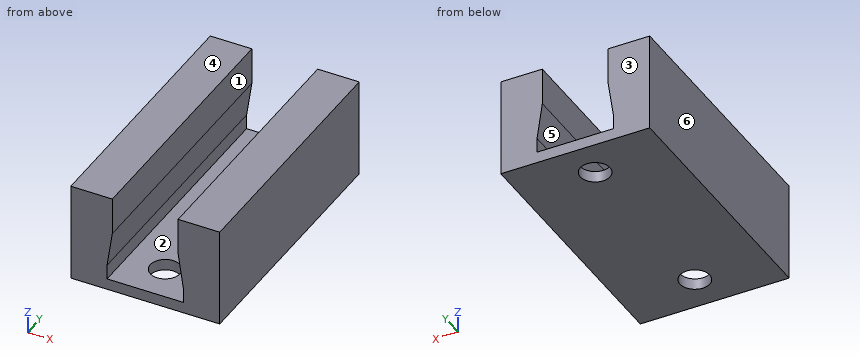
```python
from build123d import *

# Parameters (mm, degrees)
F1_DEPTH = 35
F2_R     = 2
F3_DEPTH = 8.301
F8_DEPTH = 35.001
F9_DEPTH = 5


# Not quite as in the source:
# - a feature names something its author has since deleted; it is built from what else it names


with BuildPart() as f1:
    # F0 (on Front) → F1 (new body)
    with BuildSketch(Plane.XZ):
        Polygon((10, 4.15), (4.15, 4.15), (-4.15, 4.15), (-10, 4.15), (-10, -4.15), (-4.15, -4.15), (4.15, -4.15), (10, -4.15), align=None)
        with BuildLine():
            ThreePointArc((5.15, -1.65), (4.8571067812, -2.3571067812), (4.15, -2.65))
            Line((4.15, -2.65), (-4.15, -2.65))
            ThreePointArc((-4.15, -2.65), (-4.8571067812, -2.3571067812), (-5.15, -1.65))
            Line((-5.15, -1.65), (-5.15, 1.65))
            ThreePointArc((-5.15, 1.65), (-4.8571067812, 2.3571067812), (-4.15, 2.65))
            Line((-4.15, 2.65), (4.15, 2.65))
            ThreePointArc((4.15, 2.65), (4.8571067812, 2.3571067812), (5.15, 1.65))
            Line((5.15, 1.65), (5.15, -1.65))
        make_face(mode=Mode.SUBTRACT)
        with BuildLine():
            Line((-4.15, -2.65), (4.15, -2.65))
            ThreePointArc((4.15, -2.65), (4.8571067812, -2.3571067812), (5.15, -1.65))
            Line((5.15, -1.65), (5.15, 1.65))
            ThreePointArc((5.15, 1.65), (4.8571067812, 2.3571067812), (4.15, 2.65))
            Line((4.15, 2.65), (-4.15, 2.65))
            ThreePointArc((-4.15, 2.65), (-4.8571067812, 2.3571067812), (-5.15, 1.65))
            Line((-5.15, 1.65), (-5.15, -1.65))
            ThreePointArc((-5.15, -1.65), (-4.8571067812, -2.3571067812), (-4.15, -2.65))
        make_face()
    extrude(amount=F1_DEPTH)

    # F2 (on face) → F3 (cut, through all)
    with BuildSketch(Plane.XY.offset(4.15)):
        with Locations((0, -5)):
            Circle(F2_R)
        with Locations((0, -30)):
            Circle(F2_R)
    extrude(amount=-F3_DEPTH, mode=Mode.SUBTRACT)

    # F7 (on offset) → F8 (cut, through all)
    with BuildSketch(Plane.XZ.offset(35)):
        Polygon((-5.1262229681, -2.646596171), (0, -2.646596171), (5.1262229681, -2.646596171), (5.1262229681, -0.6600963534), (4.3867812492, 4.353403829), (0, 4.353403829), (-4.3867812492, 4.353403829), (-5.1262229681, -0.6600963534), align=None)
    extrude(amount=-F8_DEPTH, mode=Mode.SUBTRACT)

    # F9 (add): faces of the model
    f9_faces = [f1.faces().sort_by_distance(p)[0] for p in [
        (-7.2083906517, -17.5, 4.15),
        (7.2083906517, -17.5, 4.15),
    ]]
    extrude(f9_faces, amount=F9_DEPTH)


solid = f1.part
```
Input: part model. Units: mm. Frame: model coordinates. Face numbers are marked on the shaded views. A direction names the side the tool comes from. Coordinates: 2 decimals unless noted, no trailing zeros. Order: outer loops, then holes, each group sorted by start corner. A loop starts at its lowest first (then second) coordinate and runs counter-clockwise, first axis right, second up. Notation, with made-up numbers: (68, 36) - (124, 36) arc R5 cw to (124, 45) - close; hole circle Ø8 at (-16.75, 14.5). An arc over 180 degrees is marked (long way). Return JSON: item names as keys, results as strings.
Q1. Cut plane B-B (z = -2). Return loops of the section in (x, y), then the cut area to 3 significant figures.
The answers:
{"outline": "(-10, -35) - (-5.13, -35) - (-5.13, 0) - (-10, 0) - close; (5.13, -35) - (10, -35) - (10, 0) - (5.13, 0) - close", "area": "341 mm2"}
Q2. Draft query along Z for the marked faces 4, 5 and 6. Return one class per face: +Z half, -Z half, draft (parallel to the pull), parting line (faces both ways), or undercut.
The answers:
{"face 4": "+Z half", "face 5": "undercut", "face 6": "draft"}
Q3. Cut plane A-A (y = -30). Return loops of the section in (x, z), then the cut area to 3 significant figures.
The answers:
{"outline": "(-10, -4.15) - (-2, -4.15) - (-2, -2.65) - (-5.13, -2.65) - (-5.13, -0.66) - (-4.42, 4.15) - (-4.42, 9.15) - (-10, 9.15) - close; (2, -4.15) - (10, -4.15) - (10, 9.15) - (4.42, 9.15) - (4.42, 4.15) - (5.13, -0.66) - (5.13, -2.65) - (2, -2.65) - close", "area": "150 mm2"}
Q4. First-contact query: pin 1 (4 mm diameter, centred on x = -4, z = 2.5, fed in from -Y). Flat tip, straight axial feed; report the tip coordinate or a pass-through.
The answers:
{"pin 1": "stops at y = -35"}
Q5. Access query for the marked faces 1, 2 and 3. Directions: +Z, -Z, +X, -X, +Y, -Y. A direction counts if a zero-diameter tool reaches every point of the face in a straight line with its end or side. Return the directions, or none.
The answers:
{"face 1": "+Z, +Y, -Y", "face 2": "+Y, -Y", "face 3": "+Z, -Z, +X, -X, +Y"}
Q6. Ray query, probe 1 along Y at (x, z) = (0, -3.25); probe 2 along X at (y, z) = (-31, -0.75); probe 3 along X at (y, z) = (-8.5, 6). Return the intervals inside material, ascending.
The answers:
{"probe 1": "y = -35 to -32, -28 to -7, -3 to 0", "probe 2": "x = -10 to -5.13, 5.13 to 10", "probe 3": "x = -10 to -4.42, 4.42 to 10"}
Q7. Cut plane D-D (y = -12). Return loops of the section in (x, z), then the cut area to 3 significant figures.
The answers:
{"outline": "(-10, -4.15) - (10, -4.15) - (10, 9.15) - (4.42, 9.15) - (4.42, 4.15) - (5.13, -0.66) - (5.13, -2.65) - (-5.13, -2.65) - (-5.13, -0.66) - (-4.42, 4.15) - (-4.42, 9.15) - (-10, 9.15) - close", "area": "156 mm2"}
Q8. Cut plane C-C (x = 0). Return loops of the section in (y, z), then the cut area to 3 significant figures.
The answers:
{"outline": "(-35, -4.15) - (-32, -4.15) - (-32, -2.65) - (-35, -2.65) - close; (-28, -4.15) - (-7, -4.15) - (-7, -2.65) - (-28, -2.65) - close; (-3, -4.15) - (0, -4.15) - (0, -2.65) - (-3, -2.65) - close", "area": "40.6 mm2"}
